Verification items for the finished model (mm, model axes). A direction names the side the tool comes from. Give positions to 0.01 mm unless a question says otherwise; leave off trailing zeros. Loops run counter-clockwise (first coordinate to the right, second up) from the corner with the lowest first, then second, coordinate; pieces in that order, holes last. Notation, with made-up numbers: (-18.75, 58) - (29.25, 58) arc R15 ccw to (29.25, 78) - close; hole circle Ø5 at (68.5, 13.5). An arc over 180 degrees is marked (long way). Use one line per item in the form item = value.
```python
from build123d import *

# Parameters (mm, degrees)
BASE_FLANGE1_DEPTH      = 38.1
CUT_EXTRUDE1_DEPTH      = 68.92188088
CUT_EXTRUDE1_DEPTH_BACK = 68.92188088
SKETCH6_R               = 2.4892
CUT_EXTRUDE2_DEPTH      = 70.01725583
FILLET1_R               = 1.5875
FILLET2_R               = 2.286


# Sheet-metal steps are written as plain solids
with BuildPart() as part:
    # Sketch1 → Base-Flange1 (new body)
    with BuildSketch(Plane.XY):
        with BuildLine():
            Line((-53.2765, -6.35), (-53.2765, 5.588))
            ThreePointArc((-53.2765, 5.588), (-53.053315367, 6.126815367), (-52.5145, 6.35))
            Line((-52.5145, 6.35), (52.5145, 6.35))
            ThreePointArc((52.5145, 6.35), (53.053315367, 6.126815367), (53.2765, 5.588))
            Line((53.2765, 5.588), (53.2765, -6.35))
            Line((53.2765, -6.35), (55.5625, -6.35))
            Line((55.5625, -6.35), (55.5625, 5.588))
            ThreePointArc((55.5625, 5.588), (54.669761469, 7.743261469), (52.5145, 8.636))
            Line((52.5145, 8.636), (-52.5145, 8.636))
            ThreePointArc((-52.5145, 8.636), (-54.669761469, 7.743261469), (-55.5625, 5.588))
            Line((-55.5625, 5.588), (-55.5625, -6.35))
            Line((-55.5625, -6.35), (-53.2765, -6.35))
        make_face()
    extrude(amount=BASE_FLANGE1_DEPTH)

    # Sketch6 → Cut-Extrude1 (cut, two sides: drawn at the far end of the back side and taken through both)
    with BuildSketch(Plane(origin=(0, 0, 0), x_dir=(0, 0, -1), z_dir=(1, 0, 0)).offset(-CUT_EXTRUDE1_DEPTH_BACK)):
        with Locations((6.35, -0.888959106)):
            Circle(SKETCH6_R)
        with Locations((-6.35, -0.888959106)):
            Circle(SKETCH6_R)
        with Locations((-19.05, -0.888959106)):
            Circle(SKETCH6_R)
        with Locations((-31.75, -0.888959106)):
            Circle(SKETCH6_R)
    extrude(amount=CUT_EXTRUDE1_DEPTH + CUT_EXTRUDE1_DEPTH_BACK, mode=Mode.SUBTRACT)

    # Sketch7 → Cut-Extrude2 (cut, through all)
    with BuildSketch(Plane(origin=(0, 8.636, 0), x_dir=(1, 0, 0), z_dir=(0, 1, 0))):
        Polygon((-26.25725, -4.806913197), (-29.08380657, -3.175), (-48.54575, -3.175), (-48.54575, -17.675184671), align=None)
        Polygon((-48.54575, -17.675184671), (-48.54575, -3.175), (-49.3395, -3.175), (-49.3395, -18.133456448), align=None)
        Polygon((-48.54575, -34.925), (-48.54575, -20.424815329), (-49.3395, -19.966543552), (-49.3395, -34.925), align=None)
        Polygon((-25.4635, -31.918271475), (-25.4635, -6.181728525), (-47.752, -19.05), align=None)
        Polygon((-27.89318157, -34.237592336), (-26.25725, -33.293086803), (-48.54575, -20.424815329), (-48.54575, -34.925), (-29.08380657, -34.925), align=None)
        Polygon((-23.876, -31.918271475), (-1.5875, -19.05), (-23.876, -6.181728525), align=None)
        Polygon((-0.79375, -17.675184671), (-0.79375, -3.175), (-20.25569343, -3.175), (-21.44631843, -3.862407664), (-23.08225, -4.806913197), align=None)
        Polygon((-0.79375, -34.925), (-0.79375, -20.424815329), (-23.08225, -33.293086803), (-21.44631843, -34.237592336), (-20.25569343, -34.925), align=None)
        Polygon((21.44631843, -3.862407664), (20.25569343, -3.175), (0.79375, -3.175), (0.79375, -17.675184671), (23.08225, -4.806913197), align=None)
        Polygon((23.876, -31.918271475), (23.876, -6.181728525), (1.5875, -19.05), align=None)
        Polygon((48.54575, -34.925), (48.54575, -20.424815329), (26.25725, -33.293086803), (27.89318157, -34.237592336), (29.08380657, -34.925), align=None)
        Polygon((25.4635, -31.918271475), (47.752, -19.05), (25.4635, -6.181728525), align=None)
        Polygon((48.54575, -17.675184671), (48.54575, -3.175), (29.08380657, -3.175), (26.25725, -4.806913197), align=None)
        Polygon((49.3395, -34.925), (49.3395, -19.966543552), (48.54575, -20.424815329), (48.54575, -34.925), align=None)
        Polygon((49.3395, -18.133456448), (49.3395, -3.175), (48.54575, -3.175), (48.54575, -17.675184671), align=None)
        Polygon((21.44631843, -34.237592336), (23.08225, -33.293086803), (0.79375, -20.424815329), (0.79375, -34.925), (20.25569343, -34.925), align=None)
    extrude(amount=-CUT_EXTRUDE2_DEPTH, mode=Mode.SUBTRACT)

    # Fillet1
    fillet1_edges = [part.edges().sort_by_distance(p)[0] for p in [
        (-20.25569343, 7.493, 34.925),
        (-23.08225, 7.493, 33.293086803),
        (-0.79375, 7.493, 20.424815329),
        (-0.79375, 7.493, 34.925),
        (20.25569343, 7.493, 3.175),
        (23.08225, 7.493, 4.806913197),
        (0.79375, 7.493, 17.675184671),
        (0.79375, 7.493, 3.175),
        (1.5875, 7.493, 19.05),
        (23.876, 7.493, 6.181728525),
        (23.876, 7.493, 31.918271475),
        (25.4635, 7.493, 31.918271475),
        (25.4635, 7.493, 6.181728525),
        (47.752, 7.493, 19.05),
        (-23.876, 7.493, 31.918271475),
        (-23.876, 7.493, 6.181728525),
        (-1.5875, 7.493, 19.05),
        (-23.08225, 7.493, 4.806913197),
        (-20.25569343, 7.493, 3.175),
        (-0.79375, 7.493, 3.175),
        (-0.79375, 7.493, 17.675184671),
        (-47.752, 7.493, 19.05),
        (-25.4635, 7.493, 6.181728525),
        (-25.4635, 7.493, 31.918271475),
        (-29.08380657, 7.493, 34.925),
        (-49.3395, 7.493, 34.925),
        (-49.3395, 7.493, 19.966543552),
        (-26.25725, 7.493, 33.293086803),
        (29.08380657, 7.493, 34.925),
        (26.25725, 7.493, 33.293086803),
        (49.3395, 7.493, 19.966543552),
        (49.3395, 7.493, 34.925),
        (26.25725, 7.493, 4.806913197),
        (29.08380657, 7.493, 3.175),
        (49.3395, 7.493, 3.175),
        (49.3395, 7.493, 18.133456448),
        (23.08225, 7.493, 33.293086803),
        (20.25569343, 7.493, 34.925),
        (0.79375, 7.493, 34.925),
        (0.79375, 7.493, 20.424815329),
        (-49.3395, 7.493, 3.175),
        (-29.08380657, 7.493, 3.175),
        (-26.25725, 7.493, 4.806913197),
        (-49.3395, 7.493, 18.133456448),
    ]]
    fillet(fillet1_edges, radius=FILLET1_R)

    # Fillet2
    fillet2_edges = [part.edges().sort_by_distance(p)[0] for p in [
        (54.4195, -6.35, 0),
        (-54.4195, -6.35, 0),
        (54.4195, -6.35, 38.1),
        (-54.4195, -6.35, 38.1),
    ]]
    fillet(fillet2_edges, radius=FILLET2_R)


solid = part.part
```
1. Tool access check on faces 1 (the flat face through (0.794, 8, 28)), 2 (the flat face through (-1, 6.35, 19)), 3 (the cylindrical face through (-54.646, 7.767, 18.783)). Record the directions out of +Z, -Z, +X, -X, +Y, -Y that give a thin tool (end or side, any length) a straight path to the whole face; none if there is none.
Result set:
face_1 = +Y, -Y
face_2 = +Z, -Z, -Y
face_3 = +Z, -Z, -X, +Y
2. Depth check by flat-ended pin: pin 1 Ø5 at (x, z) = (-34, 24) entering from +Y; pin 2 Ø2.5 at (y, z) = (7, 22.5) entering from -X; pin 3 Ø1.1 at (y, z) = (7, 19.5) entering from +X; pin 4 Ø2.5 at (y, z) = (7.5, 30.5) entering from -X. Enter the tip coordinate at first touch or a pass-through.
Result set:
pin_1 = through
pin_2 = -55.56
pin_3 = 55.44
pin_4 = -55.49
3. Section check A-A, the plane x = -17. State how many separate pieces and enclosed holes the cut face has, then the cut area to 3 significant figures.
Result set:
separate_pieces = 4
enclosed_holes = 0
area = 22.9 mm²
4. Scan lines: probe 1 along X at (y, z) = (-0.25, 25.5); probe 2 along Z at (x, y) = (-14.5, 7) (3 decimals); probe 3 along Y at (x, z) = (40, 2). Record each from-to range of solid material in increasing order.
Result set:
probe_1 = -55.56 to -53.28, 53.28 to 55.56
probe_2 = 0 to 3.175, 9.762 to 11.595, 26.505 to 28.338, 34.925 to 38.1
probe_3 = 6.35 to 8.64
5. Section check B-B, the plane y = -5.25. Record the cut outline in (x, z).
Result set:
outline = (-55.56, 0.33) - (-53.28, 0.33) - (-53.28, 37.77) - (-55.56, 37.77) - close; (53.28, 0.33) - (55.56, 0.33) - (55.56, 37.77) - (53.28, 37.77) - close
6. Draft check along Z on faces 4 (the flat face through (-37.67, 7.509, 26.704)), 5 (the cylindrical face through (54.44, -5.66, 37.45)), 6 (the cylindrical face through (54.44, -5.66, 0.65)), 7 (the flat face through (-37.927, 7.509, 11.544)). Enter one of: released by +Z, released by -Z, zero draft, split by the parting line, or undercut.
Result set:
face_4 = undercut
face_5 = released by +Z
face_6 = released by -Z
face_7 = undercut
